from build123d import *

# Parameters (mm, degrees)
AUFSATZ_LINEAR_AUSTRAGEN1_DEPTH = 6.4
SKIZZE2_W                       = 175
SKIZZE2_H                       = 80
AUFSATZ_LINEAR_AUSTRAGEN2_DEPTH = 63
VERRUNDUNG1_R                   = 5
VERRUNDUNG2_R                   = 3
SKIZZE3_R                       = 9
AUFSATZ_LINEAR_AUSTRAGEN3_DEPTH = 70
SKIZZE4_R                       = 10.5
AUFSATZ_LINEAR_AUSTRAGEN4_DEPTH = 60


with BuildPart() as part:
    # Skizze1 → Aufsatz-Linear austragen1 (new body)
    with BuildSketch(Plane(origin=(0, 0, 0), x_dir=(1, 0, 0), z_dir=(0, 1, 0))):
        with BuildLine():
            Line((-106.3, -37), (-106.3, 37))
            ThreePointArc((-106.3, 37), (-105.421320344, 39.121320344), (-103.3, 40))
            Line((-103.3, 40), (103.3, 40))
            ThreePointArc((103.3, 40), (105.421320344, 39.121320344), (106.3, 37))
            Line((106.3, 37), (106.3, -37))
            ThreePointArc((106.3, -37), (105.421320344, -39.121320344), (103.3, -40))
            Line((103.3, -40), (-103.3, -40))
            ThreePointArc((-103.3, -40), (-105.421320344, -39.121320344), (-106.3, -37))
        make_face()
        with BuildLine():
            Line((-94.4, 30.5), (-94.4, 12.7))
            ThreePointArc((-94.4, 12.7), (-97.4, 9.7), (-100.4, 12.7))
            Line((-100.4, 12.7), (-100.4, 30.5))
            ThreePointArc((-100.4, 30.5), (-97.4, 33.5), (-94.4, 30.5))
        make_face(mode=Mode.SUBTRACT)
        with BuildLine():
            Line((-94.4, -30.5), (-94.4, -12.7))
            ThreePointArc((-94.4, -12.7), (-97.4, -9.7), (-100.4, -12.7))
            Line((-100.4, -12.7), (-100.4, -30.5))
            ThreePointArc((-100.4, -30.5), (-97.4, -33.5), (-94.4, -30.5))
        make_face(mode=Mode.SUBTRACT)
        with BuildLine():
            Line((94.4, 30.5), (94.4, 12.7))
            ThreePointArc((94.4, 12.7), (97.4, 9.7), (100.4, 12.7))
            Line((100.4, 12.7), (100.4, 30.5))
            ThreePointArc((100.4, 30.5), (97.4, 33.5), (94.4, 30.5))
        make_face(mode=Mode.SUBTRACT)
        with BuildLine():
            Line((94.4, -30.5), (94.4, -12.7))
            ThreePointArc((94.4, -12.7), (97.4, -9.7), (100.4, -12.7))
            Line((100.4, -12.7), (100.4, -30.5))
            ThreePointArc((100.4, -30.5), (97.4, -33.5), (94.4, -30.5))
        make_face(mode=Mode.SUBTRACT)
    extrude(amount=AUFSATZ_LINEAR_AUSTRAGEN1_DEPTH)

    # Skizze2 → Aufsatz-Linear austragen2 (add)
    with BuildSketch(Plane(origin=(0, 6.4, 0), x_dir=(1, 0, 0), z_dir=(0, 1, 0))):
        Rectangle(SKIZZE2_W, SKIZZE2_H)
    extrude(amount=AUFSATZ_LINEAR_AUSTRAGEN2_DEPTH)

    # Verrundung1
    verrundung1_edges = [part.edges().sort_by_distance(p)[0] for p in [
        (-87.5, 37.9, 40),
        (87.5, 37.9, 40),
        (87.5, 37.9, -40),
        (-87.5, 37.9, -40),
    ]]
    fillet(verrundung1_edges, radius=VERRUNDUNG1_R)

    # Verrundung2
    verrundung2_edges = [part.edges().sort_by_distance(p)[0] for p in [
        (0, 69.4, 40),
        (-87.5, 69.4, 0),
        (86.035533906, 69.4, 38.535533906),
        (-86.035533906, 69.4, 38.535533906),
        (-86.035533906, 69.4, -38.535533906),
        (86.035533906, 69.4, -38.535533906),
        (0, 69.4, -40),
        (87.5, 69.4, 0),
    ]]
    fillet(verrundung2_edges, radius=VERRUNDUNG2_R)

    # Skizze3 → Aufsatz-Linear austragen3 (add)
    with BuildSketch(Plane(origin=(0, 0, -40), x_dir=(-1, 0, 0), z_dir=(0, 0, -1))):
        with Locations(Location((-56.2, 34, 0), (0, 0, 180))):
            Circle(SKIZZE3_R)
        with Locations(Location((16.4, 34, 0), (0, 0, 180))):
            Circle(SKIZZE3_R)
    extrude(amount=AUFSATZ_LINEAR_AUSTRAGEN3_DEPTH)

    # Skizze4 → Aufsatz-Linear austragen4 (add)
    with BuildSketch(Plane.ZY.offset(87.5)):
        with Locations(Location((0, 35.4, 0), (0, 0, 180))):
            Circle(SKIZZE4_R)
    extrude(amount=AUFSATZ_LINEAR_AUSTRAGEN4_DEPTH)


solid = part.part
For this review, take the finished solid that the model builds, in its own axes (mm). A direction names the side the tool comes from. Round coordinates to 2 decimals unless told otherwise and drop trailing zeros. Loops run counter-clockwise (first coordinate to the right, second up) from the corner with the lowest first, then second, coordinate; pieces in that order, holes last. Notation, with made-up numbers: (58.25, 66.25) - (92.25, 66.25) arc R31 cw to (92.25, 103.25) - close; hole circle Ø11 at (80, 85). An arc over 180 degrees is marked (long way). Put each result on its own line as item: value. Start each with the question number.
1. Consider section D-D on y = 10.5. State the section outline as (x, z) points, plus the area to 3 significant figures.
2. Mouldability with a two-part tool opening along Y and no side actions: class faces 5 (the cylindrical face through (97.5, 3.2, -33.5)), 6 (the flat face through (1, 0, -1)), 7 (the flat face through (97, 6.4, -1)), 8 (the flat face through (-97, 6.4, -1)) as +Y half, -Y half, draft (parallel to the pull), parting line (faces both ways), or undercut.
3. For probe 1 along X at (y, z) = (34, -51.5); probe 2 along X at (y, z) = (38.5, -34); probe 3 along Z at (x, y) = (10, 47), list the stretches that pass through material, from the lowest coordinate up. Write a range as [from, to].
4. Consider section B-B on x = 97.4. State the section outline as (y, z) points, plus the area to 3 significant figures.
5. Consider section A-A on z = -21.5. State the section outline as (x, y) points, plus the area to 3 significant figures.
6. Insertion check: P1, Ø6, axis at y = 44.5, z = -30, coming from the +X side; P2, Ø5, axis at y = 3, z = 26, coming from the -X side; P3, Ø4, axis at x = -77, y = 28.5, coming from the -Z side; P4, Ø19, axis at x = -89.5, z = 6, coming from the +Y side. Each pin has a flat end and moves straight along its axis. Give the tip position at first contact, or say it passes through.
7. For faces 1 (the cylindrical face through (-86, 36.82, -38.57)), 2 (the cylindrical face through (-97.3, 3.2, -9.7)), 3 (the flat face through (94.4, 3, -22)), 4 (the cylindrical face through (86, 36.82, -38.57)), list the 3-axis set-ups (+Z, -Z, +X, -X, +Y, -Y) from which the entire face can be reached by the end or side of a thin tool; tool diameter is ignored.
8. Consider section C-C on x = -97.4. State the section outline as (y, z) points, plus the area to 3 significant figures.
Result sheet:
1. outline: (-87.5, -35) arc R5 ccw to (-82.5, -40) - (82.5, -40) arc R5 ccw to (87.5, -35) - (87.5, 35) arc R5 ccw to (82.5, 40) - (-82.5, 40) arc R5 ccw to (-87.5, 35) - close
1. area: 14,000 mm^2
2. face 5: draft
2. face 6: -Y half
2. face 7: +Y half
2. face 8: undercut
3. probe 1: [-25.4, -7.4], [47.2, 65.2]
3. probe 2: [-87.5, 87.5]
3. probe 3: [-40, 40]
4. outline: (0, -40) - (6.4, -40) - (6.4, -33.5) - (0, -33.5) - close; (0, -9.7) - (6.4, -9.7) - (6.4, 9.7) - (0, 9.7) - close; (0, 33.5) - (6.4, 33.5) - (6.4, 40) - (0, 40) - close
4. area: 207 mm^2
5. outline: (-106.3, 0) - (-100.4, 0) - (-100.4, 6.4) - (-106.3, 6.4) - close; (-94.4, 0) - (94.4, 0) - (94.4, 6.4) - (87.5, 6.4) - (87.5, 66.4) arc R3 ccw to (84.5, 69.4) - (-84.5, 69.4) arc R3 ccw to (-87.5, 66.4) - (-87.5, 6.4) - (-94.4, 6.4) - close; (100.4, 0) - (106.3, 0) - (106.3, 6.4) - (100.4, 6.4) - close
5. area: 12,300 mm^2
6. P1: x = 87.5
6. P2: x = -106.3
6. P3: z = -40
6. P4: y = 69.4
7. face 1: -Z, -X, +Y
7. face 2: -Y
7. face 3: +Y, -Y
7. face 4: -Z, +X, +Y
8. outline: (0, -40) - (6.4, -40) - (6.4, -33.5) - (0, -33.5) - close; (0, -9.7) - (6.4, -9.7) - (6.4, 9.7) - (0, 9.7) - close; (0, 33.5) - (6.4, 33.5) - (6.4, 40) - (0, 40) - close; circle Ø21 at (35.4, 0)
8. area: 554 mm^2
